Here's how the part is built. I have some questions about the finished solid (model axes, mm). A direction names the side the tool comes from. Round coordinates to 2 decimals unless told otherwise and drop trailing zeros. Write each loop counter-clockwise with the first axis right and the second up, starting at its lowest first coordinate (ties: lowest second). Pieces come first, ordered by that corner, then holes. Notation, with made-up numbers: (79.5, 41.5) -> (110.5, 41.5) arc R16 ccw to (110.5, 69.5) -> close; hole circle Ø1 at (-5.5, 38). An arc over 180 degrees is marked (long way). Answer as CSV lines item,"result".
```python
from build123d import *

# Parameters (mm, degrees)
SKETCH2_W           = 120
SKETCH2_H           = 120
BOSS_EXTRUDE1_DEPTH = 90
FILLET1_R           = 10
SHELL1_T            = -4
CUT_EXTRUDE1_DEPTH  = 20
SKETCH4_R           = 6.35
CUT_EXTRUDE2_DEPTH  = 199.773717644


with BuildPart() as part:
    # Sketch2 → Boss-Extrude1 (new body)
    with BuildSketch(Plane.XY):
        with Locations((60, 60)):
            Rectangle(SKETCH2_W, SKETCH2_H)
    extrude(amount=BOSS_EXTRUDE1_DEPTH)

    # Fillet1
    fillet1_edges = [part.edges().sort_by_distance(p)[0] for p in [
        (0, 120, 45),
        (120, 120, 45),
        (120, 0, 45),
        (0, 0, 45),
    ]]
    fillet(fillet1_edges, radius=FILLET1_R)

    # Shell1
    shell1_openings = [part.faces().sort_by_distance(p)[0] for p in [
        (60, 60, 90),
    ]]
    offset(amount=SHELL1_T, openings=shell1_openings, kind=Kind.INTERSECTION)

    # Sketch3 → Cut-Extrude1 (cut)
    with BuildSketch(Plane.XY.offset(90)):
        with BuildLine():
            Line((0, 110), (0, 10))
            ThreePointArc((0, 10), (2.928932188, 2.928932188), (10, 0))
            Line((10, 0), (110, 0))
            ThreePointArc((110, 0), (117.071067812, 2.928932188), (120, 10))
            Line((120, 10), (120, 110))
            ThreePointArc((120, 110), (117.071067812, 117.071067812), (110, 120))
            Line((110, 120), (10, 120))
            ThreePointArc((10, 120), (2.928932188, 117.071067812), (0, 110))
        make_face()
        with BuildLine():
            Line((2.2, 110), (2.2, 10))
            ThreePointArc((2.2, 10), (4.484567107, 4.484567107), (10, 2.2))
            Line((10, 2.2), (110, 2.2))
            ThreePointArc((110, 2.2), (115.515432893, 4.484567107), (117.8, 10))
            Line((117.8, 10), (117.8, 110))
            ThreePointArc((117.8, 110), (115.515432893, 115.515432893), (110, 117.8))
            Line((110, 117.8), (10, 117.8))
            ThreePointArc((10, 117.8), (4.484567107, 115.515432893), (2.2, 110))
        make_face(mode=Mode.SUBTRACT)
    extrude(amount=-CUT_EXTRUDE1_DEPTH, mode=Mode.SUBTRACT)

    # Sketch4 → Cut-Extrude2 (cut, through all)
    with BuildSketch(Plane(origin=(92.802964226, -8.446878735, 120), x_dir=(1, 0, 0), z_dir=(0, 0, 1))):
        with Locations((-73.752964226, 109.396878735)):
            Circle(SKETCH4_R)
    extrude(amount=-CUT_EXTRUDE2_DEPTH, mode=Mode.SUBTRACT)


solid = part.part
```
1. Suppose I cut it at C-C on z = 46.5. Please give me the cut outline in (x, y).
Numbers:
outline,"(0, 10) arc R10 ccw to (10, 0) -> (110, 0) arc R10 ccw to (120, 10) -> (120, 110) arc R10 ccw to (110, 120) -> (10, 120) arc R10 ccw to (0, 110) -> close; hole (4, 10) arc R6 ccw to (10, 4) -> (110, 4) arc R6 ccw to (116, 10) -> (116, 110) arc R6 ccw to (110, 116) -> (10, 116) arc R6 ccw to (4, 110) -> close"
2. Suppose I cut it at A-A on y = 100.95. Please give me the cut outline in (x, z).
Numbers:
outline,"(0, 0) -> (12.7, 0) -> (12.7, 4) -> (4, 4) -> (4, 90) -> (2.2, 90) -> (2.2, 70) -> (0, 70) -> close; (25.4, 0) -> (120, 0) -> (120, 70) -> (117.8, 70) -> (117.8, 90) -> (116, 90) -> (116, 4) -> (25.4, 4) -> close"
3. Suppose I cut it at D-D on y = 68.5. Please give me the cut outline in (x, z), and give its area (3 significant figures).
Numbers:
outline,"(0, 0) -> (120, 0) -> (120, 70) -> (117.8, 70) -> (117.8, 90) -> (116, 90) -> (116, 4) -> (4, 4) -> (4, 90) -> (2.2, 90) -> (2.2, 70) -> (0, 70) -> close"
area,"1,080 mm^2"
4. On a 3-axis mill with a long thin cutter (end or side, diameter ignored), from which of +Z, -Z, +X, -X, +Y, -Y can I reach the whole of each face in a straight line? I mean faces 4 (the face through (4.55, 115.58, 80.14)), 5 (the face through (2.2, 61, 80)), 6 (the face through (115.45, 4.42, 80.14)), 7 (the face through (117.8, 59, 80)), 8 (the face through (59, 2.2, 80)). Say none if no direction works.
Numbers:
face 4,"+Z, -X, +Y"
face 5,"+Z, -X, +Y, -Y"
face 6,"+Z, +X, -Y"
face 7,"+Z, +X, +Y, -Y"
face 8,"+Z, +X, -X, -Y"
5. If I drill on line 1 (Y direction, x = 19, z = 1); line 2 (Y direction, x = 64, z = 38.5), over which ranges is the centre line in solid material (lowest first)?
Numbers:
line 1,"y = 0 to 94.6, 107.3 to 120"
line 2,"y = 0 to 4, 116 to 120"
6. For pin 1 Ø7.5 at (x, y) = (19.05, 100.95) entering from -Z; pin 2 Ø6 at (y, z) = (62, 79) entering from +X; pin 3 Ø6 at (y, z) = (46.5, 84.5) entering from -X; pin 4 Ø10 at (x, z) = (77.5, 83) entering from -Y, each with a flat end and sliding along its axis, tell me the tip position at first contact or that it passes through.
Numbers:
pin 1,"passes through"
pin 2,"stops at x = 117.8"
pin 3,"stops at x = 2.2"
pin 4,"stops at y = 2.2"
7. If we mould it in two halves opening along Y, with no side actions, what happens to faces 1 (the face through (4.42, 4.55, 80.14)), 2 (the face through (2.85, 116.99, 35.49)), 3 (the face through (114.196, 5.711, 47.602))? For each: released by +Y, released by -Y, zero draft, split by the parting line, or undercut.
Numbers:
face 1,"released by -Y"
face 2,"released by +Y"
face 3,"undercut"
8. Suppose I cut it at B-B on x = 19.05. Please give me the cut outline in (y, z), and give its area (3 significant figures).
Numbers:
outline,"(0, 0) -> (94.6, 0) -> (94.6, 4) -> (4, 4) -> (4, 90) -> (2.2, 90) -> (2.2, 70) -> (0, 70) -> close; (107.3, 0) -> (120, 0) -> (120, 70) -> (117.8, 70) -> (117.8, 90) -> (116, 90) -> (116, 4) -> (107.3, 4) -> close"
area,"1,030 mm^2"
